```python
from build123d import *

# Parameters (mm, degrees)
ESQUISSE1_W             = 160
ESQUISSE1_H             = 160
BOSS_EXTRU_1_DEPTH      = 5
CHANFREIN1_SIZE         = 22
ESQUISSE2_W             = 20
ESQUISSE2_H             = 40
ENL_V_MAT_EXTRU_1_DEPTH = 5
ESQUISSE3_R             = 2.5
ENL_V_MAT_EXTRU_2_DEPTH = 5
ESQUISSE4_R             = 2.5
ENL_V_MAT_EXTRU_3_DEPTH = 5
ESQUISSE5_R             = 2.5
ENL_V_MAT_EXTRU_4_DEPTH = 10
ESQUISSE6_R             = 2.5
ENL_V_MAT_EXTRU_5_DEPTH = 10
ESQUISSE7_R             = 2.5
ENL_V_MAT_EXTRU_6_DEPTH = 10
ESQUISSE8_R             = 2.5
ENL_V_MAT_EXTRU_7_DEPTH = 10
ESQUISSE9_R             = 2.5
ENL_V_MAT_EXTRU_8_DEPTH = 30
ESQUISSE10_R            = 2.5
ENL_V_MAT_EXTRU_9_DEPTH = 30


with BuildPart() as part:
    # Esquisse1 → Boss.-Extru.1 (new body)
    with BuildSketch(Plane.XY):
        with Locations((51.649882403, -45.84323181)):
            Rectangle(ESQUISSE1_W, ESQUISSE1_H)
    extrude(amount=BOSS_EXTRU_1_DEPTH)

    # Chanfrein1
    chanfrein1_edges = [part.edges().sort_by_distance(p)[0] for p in [
        (-28.350117597, 34.15676819, 2.5),
        (131.649882403, 34.15676819, 2.5),
        (131.649882403, -125.84323181, 2.5),
        (-28.350117597, -125.84323181, 2.5),
    ]]
    chamfer(chanfrein1_edges, length=CHANFREIN1_SIZE)

    # Esquisse2 → Enlèv. mat.-Extru.1 (cut)
    with BuildSketch(Plane.XY.offset(5)):
        with Locations((51.649882403, -45.84323181)):
            Rectangle(ESQUISSE2_W, ESQUISSE2_H)
    extrude(amount=-ENL_V_MAT_EXTRU_1_DEPTH, mode=Mode.SUBTRACT)

    # Esquisse3 → Enlèv. mat.-Extru.2 (cut)
    with BuildSketch(Plane.XY.offset(5)):
        with Locations((46.149882403, -20.84323181)):
            Circle(ESQUISSE3_R)
        with Locations((57.149882403, -20.84323181)):
            Circle(ESQUISSE3_R)
    extrude(amount=-ENL_V_MAT_EXTRU_2_DEPTH, mode=Mode.SUBTRACT)

    # Esquisse4 → Enlèv. mat.-Extru.3 (cut)
    with BuildSketch(Plane.XY.offset(5)):
        with Locations((46.149882403, -70.84323181)):
            Circle(ESQUISSE4_R)
        with Locations((57.149882403, -61.84323181)):
            Circle(ESQUISSE4_R)
    extrude(amount=-ENL_V_MAT_EXTRU_3_DEPTH, mode=Mode.SUBTRACT)

    # Esquisse5 → Enlèv. mat.-Extru.4 (cut)
    with BuildSketch(Plane(origin=(0, 0, 0), x_dir=(-1, 0, 0), z_dir=(0, 0, -1))):
        with Locations((-57.149882403, -70.84323181)):
            Circle(ESQUISSE5_R)
    extrude(amount=-ENL_V_MAT_EXTRU_4_DEPTH, mode=Mode.SUBTRACT)

    # Esquisse6 → Enlèv. mat.-Extru.5 (cut)
    with BuildSketch(Plane.XY.offset(5)):
        with Locations((51.649882403, 29.15676819)):
            Circle(ESQUISSE6_R)
    extrude(amount=-ENL_V_MAT_EXTRU_5_DEPTH, mode=Mode.SUBTRACT)

    # Esquisse7 → Enlèv. mat.-Extru.6 (cut)
    with BuildSketch(Plane.XY.offset(5)):
        with Locations((-23.350117597, -45.84323181)):
            Circle(ESQUISSE7_R)
    extrude(amount=-ENL_V_MAT_EXTRU_6_DEPTH, mode=Mode.SUBTRACT)

    # Esquisse8 → Enlèv. mat.-Extru.7 (cut)
    with BuildSketch(Plane.XY.offset(5)):
        with Locations((51.649882403, -120.84323181)):
            Circle(ESQUISSE8_R)
        with Locations((126.649882403, -45.84323181)):
            Circle(ESQUISSE8_R)
    extrude(amount=-ENL_V_MAT_EXTRU_7_DEPTH, mode=Mode.SUBTRACT)

    # Esquisse9 → Enlèv. mat.-Extru.8 (cut)
    with BuildSketch(Plane.XY.offset(5)):
        with Locations((111.649882403, -105.84323181)):
            Circle(ESQUISSE9_R)
        with Locations((-8.350117597, -105.84323181)):
            Circle(ESQUISSE9_R)
    extrude(amount=-ENL_V_MAT_EXTRU_8_DEPTH, mode=Mode.SUBTRACT)

    # Esquisse10 → Enlèv. mat.-Extru.9 (cut)
    with BuildSketch(Plane(origin=(0, 0, 0), x_dir=(-1, 0, 0), z_dir=(0, 0, -1))):
        with Locations((-71.649882403, -85.84323181)):
            Circle(ESQUISSE10_R)
        with Locations((-31.649882403, -85.84323181)):
            Circle(ESQUISSE10_R)
    extrude(amount=-ENL_V_MAT_EXTRU_9_DEPTH, mode=Mode.SUBTRACT)


solid = part.part
```
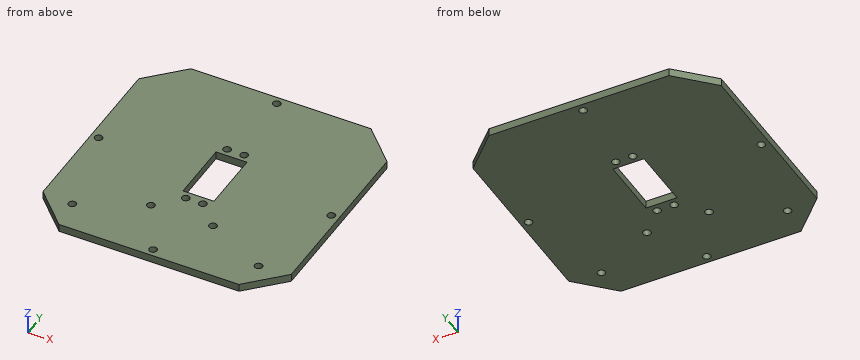
Geometry: final body of the model. Coordinates: model frame, mm. Round coordinates to 2 decimals unless told otherwise and drop trailing zeros. Order: outer loops, then holes, each group sorted by start corner. A loop starts at its lowest first (then second) coordinate and runs counter-clockwise, first axis right, second up. Notation, with made-up numbers: M 0,-26 L 18,-26 A19 cw 18,10 Z; hole C -27,31.25 d11. An arc over 180 degrees is marked long. Use one line per item in the form item = value. Start each with the question number.
Q1. Cut plane D-D (y = 17). Return loops of the section in (x, z).
Q2. Cut plane C-C (z = 3.3). Count the separate pieces of the cut face and the enclosed holes in it, and give its area (3 significant figures).
Q3. Cut plane A-A (y = -40.5). Return loops of the section in (x, z), and give its area (3 significant figures).
Q4. Cut plane B-B (x = 31.5). Return loops of the section in (y, z), and give its area (3 significant figures).
Q5. Pin query (flat end, axial travel): pin 1 Ø4 at (x, y) = (71.65, -85.84) entering from -Z; pin 2 Ø6.5 at (x, y) = (57.15, -20.84) entering from -Z; pin 3 Ø1.5 at (y, z) = (16, 3.5) entering from -X. Return the tip coordinate at first contact, or that it passes through.
Q6. Material intervals for line 1 (X direction, y = -86, z = 3.75); line 2 (X direction, y = -54.5, z = 0.5); line 3 (X direction, y = -46, z = 1.95), sorted ascending. Write a range as [from, to].
Geometry results:
q1.outline = M -23.51,0 L 126.81,0 L 126.81,5 L -23.51,5 Z
q2.separate_pieces = 1
q2.enclosed_holes = 13
q2.area = 23,600 mm^2
q3.outline = M -28.35,0 L 41.65,0 L 41.65,5 L -28.35,5 Z; M 61.65,0 L 131.65,0 L 131.65,5 L 61.65,5 Z
q3.area = 700 mm^2
q4.outline = M -125.84,0 L -88.34,0 L -88.34,5 L -125.84,5 Z; M -83.35,0 L 34.16,0 L 34.16,5 L -83.35,5 Z
q4.area = 775 mm^2
q5.pin_1 = through
q5.pin_2 = 0
q5.pin_3 = -25.26
q6.line_1 = [-28.35, 29.15], [34.14, 69.15], [74.14, 131.65]
q6.line_2 = [-28.35, 41.65], [61.65, 131.65]
q6.line_3 = [-28.35, -25.85], [-20.86, 41.65], [61.65, 124.15], [129.14, 131.65]
